Autodesk Inventor part; units mm, degrees
ref_plane "YZ Plane" through (0, 0, 0) normal (1, 0, 0) x (0, 1, 0)
ref_plane "XZ Plane" through (0, 0, 0) normal (0, 1, 0) x (-1, 0, 0)
ref_plane "XY Plane" through (0, 0, 0) normal (0, 0, 1) x (1, 0, 0)
sketch "Sketch1" plane through (0, 0, 0) normal (0, 0, 1) x (1, 0, 0)
  circle A0 centre (0, 0) radius 2.5527
  line L0 (7.3323, 0) -> (3.6662, -6.35)
  line L1 (3.6662, -6.35) -> (-3.6662, -6.35)
  line L2 (-3.6662, -6.35) -> (-7.3323, 0)
  line L3 (-7.3323, 0) -> (-3.6662, 6.35)
  line L4 (-3.6662, 6.35) -> (3.6662, 6.35)
  line L5 (3.6662, 6.35) -> (7.3323, 0)
  point P0 (0, 6.35)
  dimension "d0" = 5.1054
  dimension "d1" = 12.7
extrude "Extrusion1" add sketch "Sketch1" along normal mid plane 44.6024
thread "Thread1"
properties part number "Hex shaft 0.201 and 0.500"
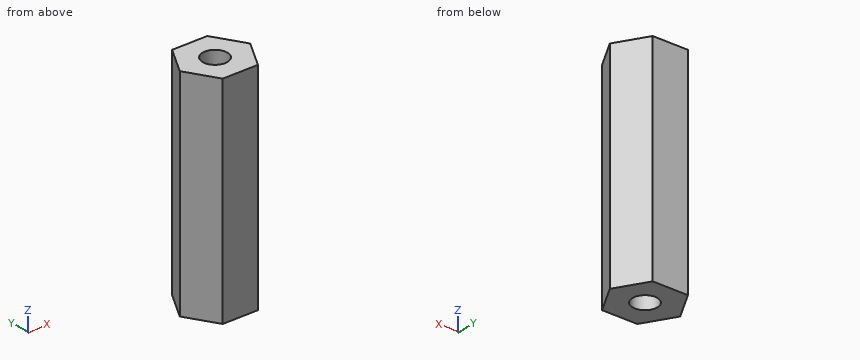
Source: CAD feature listing. Evaluate the final solid. Frame: model axes, mm. Give positions to 0.01 mm unless a question says otherwise; leave off trailing zeros. Write each loop counter-clockwise with the first axis right and the second up, starting at its lowest first coordinate (ties: lowest second). Pieces come first, ordered by that corner, then holes.
1. Section query D-D (x = 5.75). Return the cut outline in (y, z).
2. Material intervals for line 1 along Y through (x, z) = (0, 8); line 2 along X through (y, z) = (-2, 12); line 3 along X through (y, z) = (1, 18), sorted ascending.
3. Section query A-A (z = 14). Return the cut outline in (x, y).
4. Section query C-C (y = -2). Return the cut outline in (x, z), then the cut area to 3 significant figures.
5. Section query B-B (x = 0). Return the cut outline in (y, z).
6. First-contact query: pin 1 (3 mm diameter, centred on y = 2.5, z = -6, fed in from +X); pin 2 (6 mm diameter, centred on y = -4.5, z = 4, fed in from +X); pin 3 (6 mm diameter, centred on y = 1, z = -6, fed in from -X); pin 4 (3 mm diameter, centred on x = 0, y = 0, fed in from -Z) (1 decimal). Flat tips, straight axial feed; report the tip coordinate or a pass-through.
Output values:
1. outline: (-2.74, -22.3) - (2.74, -22.3) - (2.74, 22.3) - (-2.74, 22.3) - close
2. line 1: y = -6.35 to -2.55, 2.55 to 6.35
2. line 2: x = -6.18 to -1.59, 1.59 to 6.18
2. line 3: x = -6.75 to -2.35, 2.35 to 6.75
3. outline: (-7.33, 0) - (-3.67, -6.35) - (3.67, -6.35) - (7.33, 0) - (3.67, 6.35) - (-3.67, 6.35) - close; hole circle Ø5.11 at (0, 0)
4. outline: (-6.18, -22.3) - (-1.59, -22.3) - (-1.59, 22.3) - (-6.18, 22.3) - close; (1.59, -22.3) - (6.18, -22.3) - (6.18, 22.3) - (1.59, 22.3) - close
4. area: 410 mm2
5. outline: (-6.35, -22.3) - (-2.55, -22.3) - (-2.55, 22.3) - (-6.35, 22.3) - close; (2.55, -22.3) - (6.35, -22.3) - (6.35, 22.3) - (2.55, 22.3) - close
6. pin 1: stops at x = 6.75
6. pin 2: stops at x = 6.47
6. pin 3: stops at x = -7.33
6. pin 4: passes through
